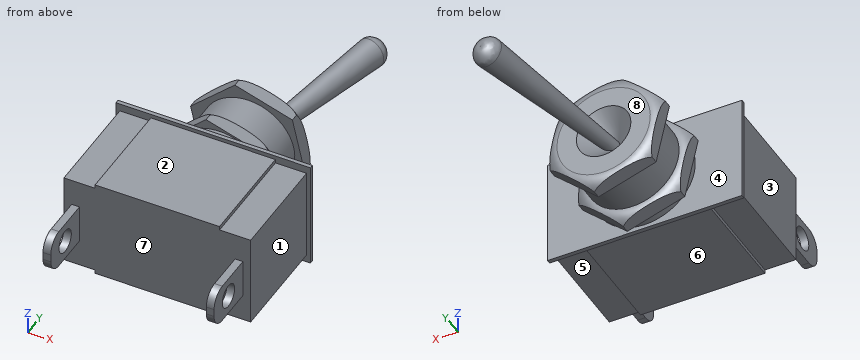
from build123d import *

# Parameters (mm, degrees)
BOSS_EXTRUDE2_DEPTH    = 13.6
SKETCH3_W              = 25
SKETCH3_H              = 14
BOSS_EXTRUDE3_DEPTH    = 0.5
SKETCH4_R              = 6
BOSS_EXTRUDE4_DEPTH    = 10
SKETCH5_R              = 6.5
BOSS_EXTRUDE5_DEPTH    = 1
SKETCH6_R              = 8
BOSS_EXTRUDE6_DEPTH    = 2
BOSS_EXTRUDE7_START    = 5
SKETCH7_R              = 8
BOSS_EXTRUDE7_DEPTH    = 2
FILLET1_R              = 1.5
FILLET2_R              = 2
CUT_EXTRUDE2_START     = -9
CUT_EXTRUDE2_OUTLINE_R = 8
CUT_EXTRUDE2_DEPTH     = 8.869095969
SKETCH13_W             = 1
SKETCH13_H             = 5
BOSS_EXTRUDE8_DEPTH    = 7
SKETCH14_R             = 1.5
CUT_EXTRUDE3_DEPTH     = 40.357608105
FILLET3_R              = 2


# Read off the part's stored shape, not the designer's step: Cut-Extrude2
with BuildPart() as part:
    # Sketch1 → Boss-Extrude2 (new body)
    with BuildSketch(Plane(origin=(0, 0, 0), x_dir=(1, 0, 0), z_dir=(0, 1, 0))):
        Polygon((-12, 6), (-8, 6), (-8, 6.5), (8, 6.5), (8, 6), (12, 6), (12, -6), (8, -6), (8, -6.5), (-8, -6.5), (-8, -6), (-12, -6), align=None)
    extrude(amount=-BOSS_EXTRUDE2_DEPTH)

    # Sketch3 → Boss-Extrude3 (add)
    with BuildSketch(Plane(origin=(0, 0, 0), x_dir=(1, 0, 0), z_dir=(0, 1, 0))):
        Rectangle(SKETCH3_W, SKETCH3_H)
    extrude(amount=BOSS_EXTRUDE3_DEPTH)

    # Sketch4 → Boss-Extrude4 (add)
    with BuildSketch(Plane(origin=(0, 0.5, 0), x_dir=(1, 0, 0), z_dir=(0, 1, 0))):
        with Locations(Location((0, 0, 0), (0, 0, 270))):
            Circle(SKETCH4_R)
    extrude(amount=BOSS_EXTRUDE4_DEPTH)

    # Sketch5 → Boss-Extrude5 (add)
    with BuildSketch(Plane(origin=(0, 0.5, 0), x_dir=(1, 0, 0), z_dir=(0, 1, 0))):
        with Locations(Location((0, 0, 0), (0, 0, 90))):
            Circle(SKETCH5_R)
    extrude(amount=BOSS_EXTRUDE5_DEPTH)

    # Sketch6 → Boss-Extrude6 (add)
    with BuildSketch(Plane(origin=(0, 1.5, 0), x_dir=(1, 0, 0), z_dir=(0, 1, 0))):
        with Locations(Location((0, 0, 0), (0, 0, 270))):
            Circle(SKETCH6_R)
    extrude(amount=BOSS_EXTRUDE6_DEPTH)

    # Sketch7 → Boss-Extrude7 (add)
    with BuildSketch(Plane(origin=(0, 3.5, 0), x_dir=(1, 0, 0), z_dir=(0, 1, 0)).offset(BOSS_EXTRUDE7_START)):
        with Locations(Location((0, 0, 0), (0, 0, 270))):
            Circle(SKETCH7_R)
    extrude(amount=BOSS_EXTRUDE7_DEPTH)

    # Cut-Extrude1 cone 1 section (through the dimple's axis) → Cut-Extrude1 (revolve, cut)
    with BuildSketch(Plane(origin=(0, 10.5, 0), x_dir=(0, 0, 1), z_dir=(1, 0, 0))):
        Polygon((0, 0), (3.5, 0), (0, 3.5), align=None)
    revolve(axis=Axis((0, 10.5, 0), (0, -1, 0)), mode=Mode.SUBTRACT)

    # Sketch8 → Revolve2 (revolve)
    with BuildSketch(Plane.XY, mode=Mode.PRIVATE) as revolve2_sk:
        Polygon((0, 5.593050937), (5.294135454, 30.5), (7.294135454, 30.5), (0.500139858, 4.447468062), align=None)
    revolve(revolve2_sk.sketch.rotate(Axis((0, 5.593050937, 0), (0.2079116908177598, 0.9781476007338056, 0)), 168.394014695), axis=Axis((0, 5.593050937, 0), (0.2079116908177598, 0.9781476007338056, 0)))

    # Fillet1
    fillet1_edges = [part.edges().sort_by_distance(p)[0] for p in [
        (7.255011561, 30.50831604, 0.393567957),
    ]]
    fillet(fillet1_edges, radius=FILLET1_R)

    # Fillet2
    fillet2_edges = [part.edges().sort_by_distance(p)[0] for p in [
        (0, 3.5, -8),
        (0, 10.5, -8),
    ]]
    fillet(fillet2_edges, radius=FILLET2_R - 0.0001)  # a hair under: the kernel refuses the full size

    # Cut-Extrude2 outline → Cut-Extrude2 (cut)
    with BuildSketch(Plane(origin=(0, 10.5, 0), x_dir=(1, 0, 0), z_dir=(0, 1, 0)).offset(CUT_EXTRUDE2_START)):
        Circle(CUT_EXTRUDE2_OUTLINE_R)
        Polygon((-1.711953383, -7.558552481), (-7.401875156, -2.296681121), (-5.689921773, 5.26187136), (1.711953383, 7.558552481), (7.401875156, 2.296681121), (5.689921773, -5.26187136), align=None, mode=Mode.SUBTRACT)
    extrude(amount=CUT_EXTRUDE2_DEPTH, mode=Mode.SUBTRACT)

    # Sketch13 → Boss-Extrude8 (add)
    with BuildSketch(Plane.XZ.offset(13.6)):
        with Locations((10.5, 0)):
            Rectangle(SKETCH13_W, SKETCH13_H)
    boss_extrude8 = extrude(amount=BOSS_EXTRUDE8_DEPTH)

    # Mirror1: Boss-Extrude8 across plane
    add(boss_extrude8.mirror(Plane(origin=(0, 0, 0), x_dir=(0, 0, 1), z_dir=(1, 0, 0))))

    # Sketch14 → Cut-Extrude3 (cut, through all)
    with BuildSketch(Plane(origin=(11, 0, 0), x_dir=(0, 0, -1), z_dir=(1, 0, 0))):
        with Locations((0, -17.1)):
            Circle(SKETCH14_R)
    extrude(amount=-CUT_EXTRUDE3_DEPTH, mode=Mode.SUBTRACT)

    # Fillet3
    fillet3_edges = [part.edges().sort_by_distance(p)[0] for p in [
        (10.5, -20.6, 2.5),
        (10.5, -20.6, -2.5),
        (-10.5, -20.6, -2.5),
        (-10.5, -20.6, 2.5),
    ]]
    fillet(fillet3_edges, radius=FILLET3_R)


solid = part.part
The model under review builds one solid part; all positions refer to its coordinate system, in mm. Face numbers are marked on the shaded views. A direction names the side the tool comes from. Round coordinates to 2 decimals unless told otherwise and drop trailing zeros. Loops run counter-clockwise (first coordinate to the right, second up) from the corner with the lowest first, then second, coordinate; pieces in that order, holes last. Notation, with made-up numbers: M -29.5,15 L 2.5,15 A15 ccw 2.5,33 Z; hole C -3,5 d11. An arc over 180 degrees is marked long. Answer as CSV lines item,"result". Start each with the question number.
Item 1: Wall thickness on line 1 (Y direction, x = -10.35, z = 0); line 2 (Y direction, x = 5.5, z = -2.5); line 3 (Y direction, x = 6.25, z = -2.25): over which ranges is each line inside the solid? List them lowest first. Write a range as [from, to].
Item 2: Insertion check: P1, Ø10, axis at x = 9, y = 0, coming from the +Z side; P2, Ø1.5, axis at y = -10.5, z = -4.5, coming from the +X side; P3, Ø4, axis at x = 9, y = 21.5, coming from the +Z side; P4, Ø2.5, axis at y = -16.5, z = 0, coming from the +X side. Each pin has a flat end and moves straight along its axis. Give the tip position at first contact, or say it passes through.
Item 3: Mouldability with a two-part tool opening along Y and no side actions: class the marked faces 6, 7 and 8 as released by +Y, released by -Y, zero draft, split by the parting line, or undercut.
Item 4: For the marked faces 1, 2, 3, 4 and 5, list the 3-axis set-ups (+Z, -Z, +X, -X, +Y, -Y) from which the entire face can be reached by the end or side of a thin tool; tool diameter is ignored.
Item 5: Consider section A-A (y = -17.1). Write out the cut boundary in (x, z).
Answer:
1,line 1,"y = [-20.6, -18.6], [-15.6, 0.5]"
1,line 2,"y = [-13.6, 3.5], [8.5, 10.5]"
1,line 3,"y = [-13.6, 0.5], [1.5, 3.39], [8.5, 10.39]"
2,P1,"stops at z = 7"
2,P2,"stops at x = 12"
2,P3,"passes through"
2,P4,"stops at x = 11"
3,face 6,"zero draft"
3,face 7,"released by -Y"
3,face 8,"undercut"
4,face 1,"+Z, -Z, +X, -Y"
4,face 2,"+Z, +X, -X, -Y"
4,face 3,"+Z, -Z, -X, -Y"
4,face 4,"none"
4,face 5,"-Z, +X, -Y"
5,outline,"M -11,-2.5 L -10,-2.5 L -10,-1.5 L -11,-1.5 Z; M -11,1.5 L -10,1.5 L -10,2.5 L -11,2.5 Z; M 10,-2.5 L 11,-2.5 L 11,-1.5 L 10,-1.5 Z; M 10,1.5 L 11,1.5 L 11,2.5 L 10,2.5 Z"
